from build123d import *

# Parameters (mm, degrees)
SKETCH1_W           = 16
SKETCH1_H           = 7
BOSS_EXTRUDE1_DEPTH = 2
SKETCH2_W           = 1.5
SKETCH2_H           = 1
CUT_EXTRUDE1_DEPTH  = 4
LPATTERN1_COUNT     = 8
LPATTERN1_PITCH     = 2.01


with BuildPart() as part:
    # Sketch1 → Boss-Extrude1 (new body)
    with BuildSketch(Plane.XY):
        with Locations((8, 3.5)):
            Rectangle(SKETCH1_W, SKETCH1_H)
    extrude(amount=BOSS_EXTRUDE1_DEPTH)

    # Sketch2 → Cut-Extrude1 (cut)
    with BuildSketch(Plane(origin=(0, 7, 0), x_dir=(1, 0, 0), z_dir=(0, 1, 0))):
        with Locations((0.95, -1)):
            Rectangle(SKETCH2_W, SKETCH2_H)
    cut_extrude1 = extrude(amount=-CUT_EXTRUDE1_DEPTH, mode=Mode.SUBTRACT)

    # LPattern1: Cut-Extrude1 ×8
    with Locations(*[(i * LPATTERN1_PITCH, 0, 0) for i in range(1, LPATTERN1_COUNT)]):
        add(cut_extrude1, mode=Mode.SUBTRACT)


solid = part.part
Work out the finished part from the listing and answer in its coordinate system (mm). A direction names the side the tool comes from. Coordinates: 2 decimals unless noted, no trailing zeros. Write each loop counter-clockwise with the first axis right and the second up, starting at its lowest first coordinate (ties: lowest second). Pieces come first, ordered by that corner, then holes. Notation, with made-up numbers: M -28.75,-1.5 L -16.75,-1.5 A28 ccw -16.75,37.5 Z; hole C 89,6.25 d4. An arc over 180 degrees is marked long. Write item = value, one per line.
1. The part is cut by section B-B (y = 3.25). State how many separate pieces and enclosed holes the cut face has, then the cut area to 3 significant figures.
Solution:
separate_pieces = 1
enclosed_holes = 8
area = 20.0 mm2
2. A flat-ended cylindrical pin translates along its axis: pin 1 (0.8 mm diameter, centred on x = 13, z = 1, fed in from +Y). Find the tip coordinate at first contact, or state that the pin passes through.
Solution:
pin_1 = 3
3. Straight lines are drawn through the part: line 1 (Z direction, x = 7, y = 5.5); line 2 (Y direction, x = 15.25, z = 0.9). For each, find the intervals that lie inside material, in ascending order. Write a range as from..to.
Solution:
line_1 = 0..0.5, 1.5..2
line_2 = 0..3
4. The part is cut by section A-A (x = 2.5). Determine the outline of the cut face in (y, z).
Solution:
outline = M 0,0 L 7,0 L 7,0.5 L 3,0.5 L 3,1.5 L 7,1.5 L 7,2 L 0,2 Z
5. Determine the mould class of faces 1 (the face through (13, 5, 1.5)), 2 (the face through (8, 0, 1)), 3 (the face through (9.74, 5, 1)) for opening direction Z: released by +Z, released by -Z, zero draft, split by the parting line, or undercut.
Solution:
face_1 = undercut
face_2 = zero draft
face_3 = undercut
6. For faces 4 (the face through (16, 3, 1)), 5 (the face through (3, 5, 0.5)), determine the directions among +Z, -Z, +X, -X, +Y, -Y from which every point of the face is accessible in a straight line to the end or side of a thin tool.
Solution:
face_4 = +Z, -Z, +X, +Y, -Y
face_5 = +Y
